Autodesk Inventor part; units mm, degrees
ref_plane "Work Plane1" through (104.775, 0, 0) normal (0, 0, -1) x (1, 0, 0)
ref_plane "YZ Plane" through (0, 0, 0) normal (1, 0, 0) x (0, 1, 0)
ref_plane "XZ Plane" through (0, 0, 0) normal (0, 1, 0) x (-1, 0, 0)
sketch "Sketch1" plane through (0, 0, 0) normal (0, 0, 1) x (1, 0, 0)
  line L0 (25, 0) -> (25, 1.5)
  line L1 (25, 1.5) -> (7, 1.5)
  line L2 (7, 1.5) -> (6.6933, 1.5)
  line L3 (0, 3) -> (0, 1.1547)
  line L4 (0, 1.1547) -> (1.05, 1.1547)
  line L5 (1.05, 1.1547) -> (1.7167, 0)
  line L6 (1.7167, 0) -> (25, 0)
  line L7 (0, 3) -> (0.36, 3)
  line L8 (0.36, 3) -> (1.86, 1.5)
  line L9 (6.6933, 1.5) -> (1.86, 1.5)
  line L10 (7, 1.5) -> (1.86, 1.5) construction
  line L11 (1.86, 1.5) -> (1.86, 1.5)
  line L12 (-5, 0) -> (30, 0)
  line L13 (0, -0.6) -> (0, 3.6)
  dimension "d0" = 25
  dimension "d1" = 18
  dimension "d2" = 1.05
  dimension "d3" = 3
  dimension "d6" = 1.86
  dimension "d7" = 45
  dimension "d8" = 2.3094
  dimension "d9" = 60
  dimension "d10" = 6
  dimension "d11" = 3
  dimension "d12" = 0.3067
revolve "Body" add sketch "Sketch1" angle 360 about axis through (1.7167, 0, 0) along (1, 0, 0) contours L6 L5 L4 L3 L7 L8 L9 L2 L1 L0
sketch "Sketch2" plane through (0, 0, 0) normal (-1, 0, 0) x (0, 0, 1)
  circle A0 centre (0, 0) radius 1.1547
  line L0 (0, -4.2) -> (0, 4.2)
  line L1 (-4.2, 0) -> (4.2, 0)
  line L2 (1.1547, 0) -> (0.5774, -1)
  line L3 (0.5774, -1) -> (-0.5774, -1)
  line L4 (-0.5774, -1) -> (-1.1547, 0)
  line L5 (-1.1547, 0) -> (-0.5774, 1)
  line L6 (-0.5774, 1) -> (0.5774, 1)
  line L7 (0.5774, 1) -> (1.1547, 0)
  point P0 (0, 1.1547)
extrude "Slot" add sketch "Sketch2" against normal up to next contours L7 A0 | A0 L2 | L6 L0 A0 | A0 L0 L3 | L0 L6 A0 | A0 L3 L0 | L4 A0 | A0 L5
thread "Thread"
chamfer "Chamfer1" distance 0.3067 distance2 0.3067 1 edges at (25, -1.5, 0) measured on face at (25, 0.0871, 0.3876)
ref_plane "Work Plane1" through (104.775, 0, 0) normal (0, 0, -1) x (1, 0, 0)
equation "\"d15\" = GEL"
equation "\"d17\" = -0.5 * SPD + 0.5 * GD"
equation "\"d18\" = GUL"
equation "\"d0\" = NLG"
equation "\"d1\" = GEL"
equation "\"d2\" = INTI"
equation "\"d3\" = GD"
equation "\"d6\" = KOH"
equation "\"d7\" = 0.5 * SEWI"
equation "\"d8\" = 1.1547 * SW"
equation "\"d10\" = KOD"
equation "\"d11\" = BDM"
equation "\"d12\" = GAL"
equation "\"NLG\" = 25"
equation "\"INTI\" = 1.05"
equation "\"GEL\" = 18"
equation "\"GAL\" = 0.61345 * PTC"
equation "\"KOH\" = 1.86"
equation "\"KOD\" = 6"
equation "\"GUL\" = 0.61345 * PTC"
equation "\"SPD\" = NND - 1.2269 * PTC"
equation "\"BDM\" = NND"
equation "\"GD\" = NND"
equation "\"SEWI\" = 90deg"
equation "\"SW\" = 2"
equation "\"TOA\" = 30deg"
equation "\"GD1\" = THREADDIA - 1.2269 * PTC"
equation "\"EPV\" = 3.36"
equation "\"THREADDIA\" = 3"
equation "\"PTC\" = 0.5"
equation "\"NND\" = 3"
equation "\"E0\" = 1.155 * SW"
properties part number "BS 4168 - M3 x 25" material "Steel, Mild"
Can you work these out from the model? Positions are in its coordinate system, mm. A direction names the side the tool comes from. Give positions to 0.01 mm unless a question says otherwise; leave off trailing zeros. Order: outer loops, then holes, each group sorted by start corner. A loop starts at its lowest first (then second) coordinate and runs counter-clockwise, first axis right, second up. Notation, with made-up numbers: (21, 37) - (60, 37) arc R23 ccw to (60, 46) - close; hole circle Ø6 at (1.25, -21). An arc over 180 degrees is marked (long way). Use a Markdown table: item, result. Add a question column.
Q1. Please list where these lines run through material, in increasing order: line 1 along X through (y, z) = (0.2, 2.2); line 2 along Z through (x, y) = (11.75, -0.95); line 3 along Y through (x, z) = (17, 0.1).
Q2. I'm going to push flat-ended pins straight in: pin 1 (1.5 mm diameter, centred on x = 15.5, z = 0.5, fed in from -Y); pin 2 (1.5 mm diameter, centred on x = 20.5, y = 1.5, fed in from -Z); pin 3 (1 mm diameter, centred on x = 5, z = 1.5, fed in from +Y). Where does each tip first touch, or does it pass through?
Q3. If we section it at A-A on x = 8: Write out the boundary of the cut face in (y, z).
Q4. If we mould it in two halves opening along Z, with no side actions, what happens to faces 4 (the flat face through (0.56, 0.51, 0.86)), 5 (the cylindrical face through (0.2, -3, 0.1)), 6 (the flat face through (0, -1.3, 0))? For each: released by +Z, released by -Z, zero draft, split by the parting line, or undercut.
Q5. On a 3-axis mill with a long thin cutter (end or side, diameter ignored), from which of +Z, -Z, +X, -X, +Y, -Y can I reach the whole of each face in a straight line? I mean faces 1 (the flat face through (25, 0, 0)), 2 (the cylindrical face through (13.12, -1.5, -0.07)), 3 (the flat face through (0.6, -1, 0)). Say none if no direction works.
Answers follow:
| question | item | result |
|---|---|---|
| 1 | line 1 | x = 0 to 1.15 |
| 1 | line 2 | z = -1.16 to 1.16 |
| 1 | line 3 | y = -1.5 to 1.5 |
| 2 | pin 1 | stops at y = -1.5 |
| 2 | pin 2 | stops at z = -1.3 |
| 2 | pin 3 | stops at y = 1.12 |
| 3 | outline | circle Ø3 at (0, 0) |
| 4 | face 4 | undercut |
| 4 | face 5 | split by the parting line |
| 4 | face 6 | zero draft |
| 5 | face 1 | +Z, -Z, +X, +Y, -Y |
| 5 | face 2 | +X |
| 5 | face 3 | -X |
